Check sheet for the modelled part. Datum: model origin and axes. Units: mm. Give positions to 0.01 mm unless a question says otherwise; leave off trailing zeros. Order: outer loops, then holes, each group sorted by start corner. A loop starts at its lowest first (then second) coordinate and runs counter-clockwise, first axis right, second up.
from build123d import *

# Parameters (mm, degrees)
SKETCH_1_R          = 4
EXTRUDE_1_DEPTH     = 3
SKETCH_2_R          = 1.5
CUT_EXTRUDE_1_DEPTH = 4
EXTRUDE_2_DEPTH     = 3
CUT_EXTRUDE_2_REACH = 5
SKETCH_4_R          = 1.6


with BuildPart() as part:
    # 草图1 → 凸台-拉伸1 (new body)
    with BuildSketch(Plane.XY):
        Polygon((90, 0), (-90, 0), (-90, -15), (-115, -15), (-115, 0), (-105, 0), (-105, 20), (105, 20), (105, 0), (115, 0), (115, -15), (90, -15), align=None)
        with Locations((0, 10)):
            Circle(SKETCH_1_R, mode=Mode.SUBTRACT)
    extrude(amount=EXTRUDE_1_DEPTH)

    # 草图2 → 切除-拉伸1 (cut, through all)
    with BuildSketch(Plane.XY.offset(3)):
        with Locations((-88.5, 0)):
            Circle(SKETCH_2_R)
        with Locations((88.5, 0)):
            Circle(SKETCH_2_R)
    extrude(amount=-CUT_EXTRUDE_1_DEPTH, mode=Mode.SUBTRACT)

    # 草图3 → 凸台-拉伸2 (add)
    with BuildSketch(Plane.XY.offset(3)):
        Polygon((-115, 0), (-105, 20), (-105, 0), align=None)
        Polygon((105, 20), (105, 0), (115, 0), align=None)
    extrude(amount=-EXTRUDE_2_DEPTH)

    # 草图4 → 切除-拉伸2 (cut, up to next)
    with BuildSketch(Plane.XY.offset(3), mode=Mode.PRIVATE) as cut_extrude_2_sk1:
        with Locations((-99.5, -7.5)):
            Circle(SKETCH_4_R)
    cut_extrude_2_tool1 = extrude(cut_extrude_2_sk1.sketch, amount=-CUT_EXTRUDE_2_REACH, mode=Mode.PRIVATE) & part.part
    add(cut_extrude_2_tool1.solids().sort_by_distance((-99.5, -7.5, 3))[0], mode=Mode.SUBTRACT)
    # 草图4 → 切除-拉伸2 (cut, up to next)
    with BuildSketch(Plane.XY.offset(3), mode=Mode.PRIVATE) as cut_extrude_2_sk2:
        with Locations((99.5, -7.5)):
            Circle(SKETCH_4_R)
    cut_extrude_2_tool2 = extrude(cut_extrude_2_sk2.sketch, amount=-CUT_EXTRUDE_2_REACH, mode=Mode.PRIVATE) & part.part
    add(cut_extrude_2_tool2.solids().sort_by_distance((99.5, -7.5, 3))[0], mode=Mode.SUBTRACT)


solid = part.part
1) Material ranges on L1, parallel to Y at x = 0, z = 1.9; L2, parallel to X at y = -4, z = 2.1; L3, parallel to Y at x = 52, z = 0.7, recorded low to high.
Recorded:
L1: y = 0 to 6, 14 to 20
L2: x = -115 to -90, 90 to 115
L3: y = 0 to 20
2) Depth check by flat-ended pin: pin 1 Ø3 at (x, y) = (-58, 9.5) entering from -Z; pin 2 Ø0.9 at (x, z) = (-25.5, 1.5) entering from -Y; pin 3 Ø1 at (y, z) = (9.5, 1.5) entering from -X. Enter the tip coordinate at first touch or a pass-through.
Recorded:
pin 1: stops at z = 0
pin 2: stops at y = 0
pin 3: stops at x = -110.5
3) Section check B-B, the plane z = 2.55. Record the cut outline in (x, y), then the cut area to 3 significant figures.
Recorded:
outline: (-115, -15) - (-90, -15) - (-90, 0) arc R1.5 cw to (-87, 0) - (87, 0) arc R1.5 cw to (90, 0) - (90, -15) - (115, -15) - (115, 0) - (105, 20) - (-105, 20) - (-115, 0) - close; hole circle Ø3.2 at (-99.5, -7.5); hole circle Ø8 at (0, 10); hole circle Ø3.2 at (99.5, -7.5)
area: 5,080 mm2
4) Draft check along Y on faces 1 (the face through (-110, 10, 2)), 2 (the face through (2, 3, 0)), 3 (the face through (-0.521, 13.966, 1.479)). Enter one of: +Y half, -Y half, draft (parallel to the pull), parting line (faces both ways), or undercut.
Recorded:
face 1: +Y half
face 2: draft
face 3: undercut
5) Section check C-C, the plane x = -11. Record the cut outline in (y, z).
Recorded:
outline: (0, 0) - (20, 0) - (20, 3) - (0, 3) - close
6) Section check A-A, the plane y = 10. Record the cut outline in (x, z), then the cut area to 3 significant figures.
Recorded:
outline: (-110, 0) - (-4, 0) - (-4, 3) - (-110, 3) - close; (4, 0) - (110, 0) - (110, 3) - (4, 3) - close
area: 636 mm2
